The listing builds one solid part. Answer for the finished solid, in the listing's coordinates (mm). Face numbers are marked on the shaded views. A direction names the side the tool comes from. Give positions to 0.01 mm unless a question says otherwise; leave off trailing zeros. Write each loop counter-clockwise with the first axis right and the second up, starting at its lowest first coordinate (ties: lowest second). Pieces come first, ordered by that corner, then holes. Notation, with made-up numbers: (75.5, -3.75) - (79.5, -3.75) arc R20 cw to (79.5, 19.25) - close; hole circle Ø3 at (-15, 41.25). An arc over 180 degrees is marked (long way). Answer in a Markdown table with one row per item. Add a question column.
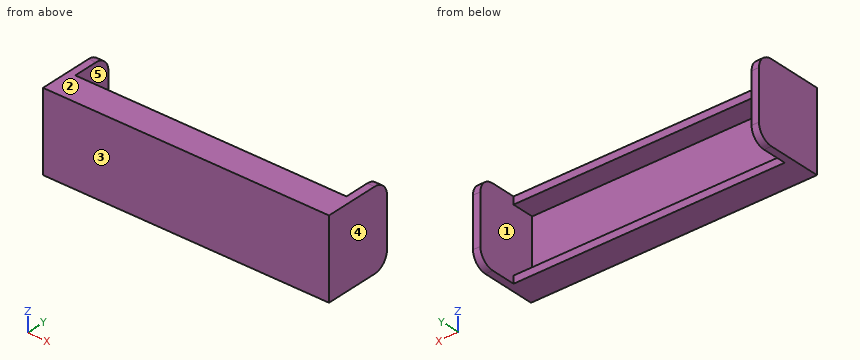
from build123d import *

# Parameters (mm, degrees)
BOSS_EXTRUDE1_DEPTH     = 29
CUT_EXTRUDE1_DEPTH      = 34.181320046
CUT_EXTRUDE1_DEPTH_BACK = 34.181320046
SKETCH4_W               = 55
SKETCH4_H               = 16
SKETCH5_W               = 55
SKETCH5_H               = 13
CUT_EXTRUDE2_DEPTH      = 4.5


with BuildPart() as part:
    # Sketch3 → Boss-Extrude1 (new, symmetric)
    with BuildSketch(Plane(origin=(0, 0, 0), x_dir=(0, 0, -1), z_dir=(1, 0, 0))):
        with BuildLine():
            Line((-8, 0), (8, 0))
            Line((8, 0), (8, 11))
            ThreePointArc((8, 11), (7.121320344, 13.121320344), (5, 14))
            Line((5, 14), (-5, 14))
            ThreePointArc((-5, 14), (-7.121320344, 13.121320344), (-8, 11))
            Line((-8, 11), (-8, 0))
        make_face()
    extrude(amount=BOSS_EXTRUDE1_DEPTH, both=True)

    # Sketch4 → Cut-Extrude1 (cut, two sides: drawn at the far end of the back side and taken through both)
    with BuildSketch(Plane.XY.offset(-CUT_EXTRUDE1_DEPTH_BACK)):
        with Locations((0, 14)):
            Rectangle(SKETCH4_W, SKETCH4_H)
    extrude(amount=CUT_EXTRUDE1_DEPTH + CUT_EXTRUDE1_DEPTH_BACK, mode=Mode.SUBTRACT)

    # Sketch5 → Cut-Extrude2 (cut)
    with BuildSketch(Plane(origin=(0, 6, 0), x_dir=(1, 0, 0), z_dir=(0, 1, 0))):
        Rectangle(SKETCH5_W, SKETCH5_H)
    extrude(amount=-CUT_EXTRUDE2_DEPTH, mode=Mode.SUBTRACT)


solid = part.part
1. A tool of negligible diameter and unlimited length cuts with its end or side. For the marked faces 1 and 2, from which of +Z, -Z, +X, -X, +Y, -Y can it reach the whole face along a straight path? Write none if from no direction.
2. Section D-D (z = 0) is taken. Give the vertices of the cut face in (x, y).
3. Given pin 1 Ø0.8 at (x, z) = (-12.5, 7) entering from +Y; pin 2 Ø1 at (x, z) = (23, -0.5) entering from +Y, each flat-ended and moving along its own axis, determine where each tip first touches the part or whether it passes through.
4. Section A-A (y = 4.75) is taken. Give the vertices of the cut face in (x, z).
5. Section B-B (y = 10.5) is taken. Give the vertices of the cut face in (x, z), and give its area (3 significant figures).
6. The mould has two halves that part along X. Classify the marked faces 3, 4 and 5: +X half, -X half, draft (parallel to the pull), parting line (faces both ways), or undercut.
7. Straight lines are drawn through the part: L1, parallel to X at y = 8.75, z = -2.5; L2, parallel to Z at x = 13.5, y = 2; L3, parallel to Y at x = 6, z = -3.5. For each, find the intervals that lie inside material, in ascending order. Write a range as [from, to].
8. Section C-C (x = 3.5) is taken. Give the vertices of the cut face in (y, z).
Geometry check:
| question | item | result |
|---|---|---|
| 1 | face 1 | +Y |
| 1 | face 2 | +Z, +X, -X, +Y, -Y |
| 2 | outline | (-29, 0) - (29, 0) - (29, 14) - (27.5, 14) - (27.5, 1.5) - (-27.5, 1.5) - (-27.5, 14) - (-29, 14) - close |
| 3 | pin 1 | y = 6 |
| 3 | pin 2 | y = 1.5 |
| 4 | outline | (-29, -8) - (29, -8) - (29, 8) - (-29, 8) - close; hole (-27.5, -6.5) - (27.5, -6.5) - (27.5, 6.5) - (-27.5, 6.5) - close |
| 5 | outline | (-29, -8) - (-27.5, -8) - (-27.5, 8) - (-29, 8) - close; (27.5, -8) - (29, -8) - (29, 8) - (27.5, 8) - close |
| 5 | area | 48.0 mm² |
| 6 | face 3 | draft |
| 6 | face 4 | +X half |
| 6 | face 5 | undercut |
| 7 | L1 | [-29, -27.5], [27.5, 29] |
| 7 | L2 | [-8, -6.5], [6.5, 8] |
| 7 | L3 | [0, 1.5] |
| 8 | outline | (0, -8) - (6, -8) - (6, -6.5) - (1.5, -6.5) - (1.5, 6.5) - (6, 6.5) - (6, 8) - (0, 8) - close |
